For this review, take the finished solid that the model builds, in its own axes (mm). Face numbers are marked on the shaded views. A direction names the side the tool comes from. Round coordinates to 2 decimals unless told otherwise and drop trailing zeros. Order: outer loops, then holes, each group sorted by start corner. A loop starts at its lowest first (then second) coordinate and runs counter-clockwise, first axis right, second up. Notation, with made-up numbers: M -1.75,-20 L 56.25,-20 A16 ccw 56.25,-15 Z; hole C 70,87.25 d3. An arc over 180 degrees is marked long. Answer in a Markdown table with one row per item. Add a question column.
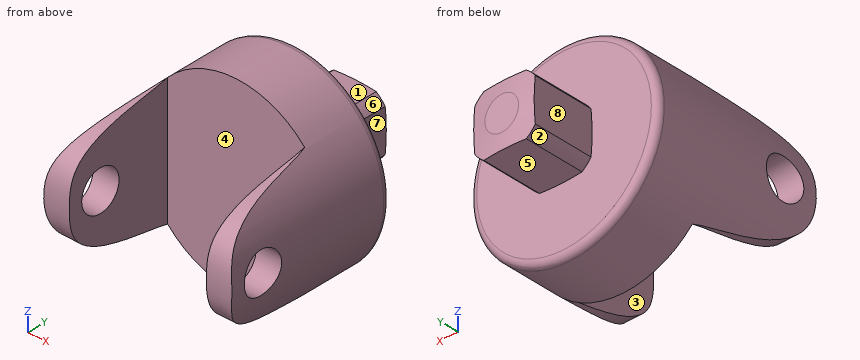
```python
from build123d import *

# Parameters (mm, degrees)
BOSS_EXTRUDE1_DEPTH      = 102
BOSS_EXTRUDE1_DEPTH_BACK = 30
SKETCH1_R                = 70
SKETCH2_W                = 45
SKETCH2_H                = 45
BOSS_EXTRUDE2_DEPTH      = 50
FILLET1_R                = 5
FILLET2_R                = 5
SKETCH4_W                = 102
SKETCH4_H                = 150
CUT_EXTRUDE1_DEPTH       = 84
CUT_EXTRUDE3_DEPTH       = 72
CUT_EXTRUDE4_DEPTH       = 182.394597571
CUT_EXTRUDE4_DEPTH_BACK  = 182.394597571
SKETCH6_R                = 15


with BuildPart() as part:
    # Sketch1 → Boss-Extrude1 (new, two sides: drawn at the far end of the back side and taken through both)
    with BuildSketch(Plane(origin=(0, 0, 0), x_dir=(1, 0, 0), z_dir=(0, 1, 0)).offset(-BOSS_EXTRUDE1_DEPTH_BACK)):
        with Locations(Location((0, 0, 0), (0, 0, 270))):
            Circle(SKETCH1_R)
    extrude(amount=BOSS_EXTRUDE1_DEPTH + BOSS_EXTRUDE1_DEPTH_BACK)

    # Sketch2 → Boss-Extrude2 (add)
    with BuildSketch(Plane(origin=(0, 102, 0), x_dir=(1, 0, 0), z_dir=(0, 1, 0))):
        Rectangle(SKETCH2_W, SKETCH2_H)
    extrude(amount=BOSS_EXTRUDE2_DEPTH)

    # Fillet1
    fillet1_edges = [part.edges().sort_by_distance(p)[0] for p in [
        (0, 102, -70),
    ]]
    fillet(fillet1_edges, radius=FILLET1_R)

    # Fillet2
    fillet2_edges = [part.edges().sort_by_distance(p)[0] for p in [
        (0, -30, -70),
    ]]
    fillet(fillet2_edges, radius=FILLET2_R)

    # Sketch3 → Cut-Revolve2 (revolve, cut)
    with BuildSketch(Plane.XY, mode=Mode.PRIVATE) as cut_revolve2_sk:
        Polygon((-12.5, 152), (-47.512769581, 152), (-47.512769581, 102), (-12.5, 102), (-27.5, 104.644904711), (-27.5, 149.355095289), align=None)
    revolve(cut_revolve2_sk.sketch.rotate(Axis((0, 160.85, 0), (0, -1, 0)), 270), axis=Axis((0, 160.85, 0), (0, -1, 0)), mode=Mode.SUBTRACT)

    # Sketch4 → Cut-Extrude1 (cut)
    with BuildSketch(Plane.XZ.offset(30)):
        Rectangle(SKETCH4_W, SKETCH4_H)
    extrude(amount=-CUT_EXTRUDE1_DEPTH, mode=Mode.SUBTRACT)

    # Sketch5 → Cut-Extrude3 (cut, symmetric)
    with BuildSketch(Plane(origin=(0, 0, 0), x_dir=(0, 0, -1), z_dir=(1, 0, 0))):
        with BuildLine():
            Line((-47.947888379, 54), (-70, 54))
            Line((-70, 54), (-70, -34.210439424))
            Line((-70, -34.210439424), (78.024892387, -34.210439424))
            Line((78.024892387, -34.210439424), (78.024892387, 54))
            Line((78.024892387, 54), (47.947888379, 54))
            add(Edge.make_bspline(
                [(47.947888379, 54), (43.174062714, 36.113920215), (41.307491939, -20.223592095), (8.979551546, -25), (0, -25)],
                knots=[0, 0, 0, 0, 0.785107117, 1, 1, 1, 1], degree=3))
            add(Edge.make_bspline(
                [(-47.947888379, 54), (-43.174062714, 36.113920215), (-41.307491939, -20.223592095), (-8.979551546, -25), (0, -25)],
                knots=[0, 0, 0, 0, 0.785107117, 1, 1, 1, 1], degree=3))
        make_face()
    extrude(amount=CUT_EXTRUDE3_DEPTH, both=True, mode=Mode.SUBTRACT)

    # Sketch6 → Cut-Extrude4 (cut, two sides: drawn at the far end of the back side and taken through both)
    with BuildSketch(Plane(origin=(0, 0, 0), x_dir=(0, 0, -1), z_dir=(1, 0, 0)).offset(-CUT_EXTRUDE4_DEPTH_BACK)):
        Circle(SKETCH6_R)
    extrude(amount=CUT_EXTRUDE4_DEPTH + CUT_EXTRUDE4_DEPTH_BACK, mode=Mode.SUBTRACT)


solid = part.part
```
1. Consider section A-A on x = 0. Write out the cut boundary in (y, z), plus the area to 3 significant figures.
2. Consider section C-C on y = 57.5. Write out the cut boundary in (x, z), plus the area to 3 significant figures.
3. Clearance check with flat-ended pins moving along their axes: pin 1 Ø8 at (x, y) = (-22, 104) entering from -Z; pin 2 Ø2 at (x, z) = (44, 8) entering from +Y; pin 3 Ø12 at (y, z) = (84.5, -13) entering from -X. State where each tip first meets the part, or that it passes through.
4. For the marked faces 4, 5, 6, 7 and 8, list the 3-axis set-ups (+Z, -Z, +X, -X, +Y, -Y) from which the entire face can be reached by the end or side of a thin tool; tool diameter is ignored.
5. To check wall thickness, follow probe 1 along Y at (x, z) = (60, 0); probe 2 along Y at (x, z) = (9.5, -37.5); probe 3 along Z at (x, y) = (62.75, 0). State the ranges of each line that lie inside material, in increasing order. Write a range as [from, to].
6. The part is to be moulded in two halves that separate along X. For the marked faces 1, 2 and 3, say which applies: pulls with the +X half, pulls with the -X half, needs draft (parallel to the pull), parting line crosses it, or undercut.
7. Consider section B-B on z = 0. State how many separate pieces and enclosed holes the cut face has, plus the area to 3 significant figures.
Solved:
| question | item | result |
|---|---|---|
| 1 | outline | M 54,-70 L 97,-70 A5 ccw 102,-65 L 102,-12.5 L 103.76,-22.5 L 150.24,-22.5 L 152,-12.5 L 152,12.5 L 150.24,22.5 L 103.76,22.5 L 102,12.5 L 102,65 A5 ccw 97,70 L 54,70 Z |
| 1 | area | 8,920 mm^2 |
| 2 | outline | C 0,0 d140 |
| 2 | area | 15,400 mm^2 |
| 3 | pin 1 | stops at z = -65.64 |
| 3 | pin 2 | stops at y = 102 |
| 3 | pin 3 | stops at x = -69.65 |
| 4 | face 4 | +Z, -Z, -Y |
| 4 | face 5 | -Z, +X, -X, +Y |
| 4 | face 6 | +Z, +X, +Y |
| 4 | face 7 | +Z, -Z, +X, +Y |
| 4 | face 8 | +Z, -Z, -X, +Y |
| 5 | probe 1 | y = [-25, -15], [15, 102] |
| 5 | probe 2 | y = [54, 102] |
| 5 | probe 3 | z = [-31.02, -15], [15, 31.02] |
| 6 | face 1 | needs draft |
| 6 | face 2 | pulls with the -X half |
| 6 | face 3 | undercut |
| 7 | separate pieces | 3 |
| 7 | enclosed holes | 0 |
| 7 | area | 10,800 mm^2 |
